Check sheet for the modelled part. Datum: model origin and axes. Units: mm. A direction names the side the tool comes from. Give positions to 0.01 mm unless a question says otherwise; leave off trailing zeros. Write each loop counter-clockwise with the first axis right and the second up, starting at its lowest first coordinate (ties: lowest second). Pieces come first, ordered by that corner, then holes. Notation, with made-up numbers: M -9.75,75 L 21.25,75 A21 cw 21.25,105 Z; hole C -21,54.5 d10. An arc over 180 degrees is marked long. Write item = value, one per line. Start each with the question number.
1) Sectioned sample at A-A, the plane z = -12. Record the cut outline in (x, y), then the cut area to 3 significant figures.
2) Scan lines: L1, parallel to X at y = 2.15, z = -4; L2, parallel to Z at x = 10.25, y = 1.5; L3, parallel to X at y = 0.3, z = -7.5. Record each from-to range of solid material in increasing order.
3) Gauge pin test, flat ends, axial feed: pin 1 (3 mm diameter, centred on x = 8, z = -10, fed in from +Y); pin 2 (0.5 mm diameter, centred on x = 12, z = -12, fed in from -Y); pin 3 (3 mm diameter, centred on x = 7, z = -3.5, fed in from -Y). Record the tip position at first contact, or that the pin passes through.
4) Draft check along X on faces 4 (the face through (4.78, 2.39, -11.83)), 5 (the face through (15, 0, -8)), 6 (the face through (4, 3.2, -4)), 7 (the face through (16, 2, -8)). Enter one of: pulls with the +X half, pulls with the -X half, needs draft (parallel to the pull), parting line crosses it, or undercut.
5) Sectioned sample at D-D, the plane y = 0.45. Record the cut outline in (x, z), then the cut area to 3 significant figures.
6) Sectioned sample at C-C, the plane x = 7.5. Record the cut outline in (y, z), then the cut area to 3 significant figures.
7) Set-up check for faces 1 (the face through (12, 4.8, -4)), 2 (the face through (3.28, 3.99, -6.29)), 3 (the face through (8, 1.6, -8)): record each of +Z, -Z, +X, -X, +Y, -Y from which the full face is reachable in a straight line by a thin tool's end or side.
8) Sectioned sample at B-B, the plane y = 2.5. Record the cut outline in (x, z), then the cut area to 3 significant figures.
from build123d import *

# Parameters (mm, degrees)
SKETCH1_W            = 16
SKETCH1_H            = 16
BOSS_EXTRUDE1_DEPTH  = 3.2
SKETCH2_R            = 2.4
BOSS_EXTRUDE2_DEPTH  = 1.6
LPATTERN1_COUNT      = 2
LPATTERN1_PITCH      = 8
LPATTERN1_COUNT_DIR2 = 4
LPATTERN1_PITCH_DIR2 = 8
SHELL1_T             = -1.6


with BuildPart() as part:
    # Sketch1 → Boss-Extrude1 (new body)
    with BuildSketch(Plane(origin=(0, 0, 0), x_dir=(1, 0, 0), z_dir=(0, 1, 0))):
        with Locations((8, 8)):
            Rectangle(SKETCH1_W, SKETCH1_H)
    extrude(amount=BOSS_EXTRUDE1_DEPTH)

    # Sketch2 → Boss-Extrude2 (add)
    with BuildSketch(Plane(origin=(0, 3.2, 0), x_dir=(1, 0, 0), z_dir=(0, 1, 0))):
        with Locations(Location((12, 4, 0), (0, 0, 90))):
            Circle(SKETCH2_R)
    boss_extrude2 = extrude(amount=BOSS_EXTRUDE2_DEPTH)

    # LPattern1: Boss-Extrude2 2 × 4, 4 skipped
    with Locations(*[(-i * LPATTERN1_PITCH, 0, -j * LPATTERN1_PITCH_DIR2) for i in range(LPATTERN1_COUNT) for j in range(LPATTERN1_COUNT_DIR2) if (i, j) not in ((0, 0), (0, 2), (0, 3), (1, 2), (1, 3))]):
        add(boss_extrude2)

    # Shell1
    shell1_openings = [part.faces().sort_by_distance(p)[0] for p in [
        (8, 0, -8),
    ]]
    offset(amount=SHELL1_T, openings=shell1_openings, kind=Kind.INTERSECTION)


solid = part.part
Data:
q1.outline = M 0,0 L 1.6,0 L 1.6,1.6 L 3.2,1.6 L 3.2,3.2 L 4.8,3.2 L 4.8,1.6 L 11.2,1.6 L 11.2,3.2 L 12.8,3.2 L 12.8,1.6 L 14.4,1.6 L 14.4,0 L 16,0 L 16,3.2 L 14.4,3.2 L 14.4,4.8 L 9.6,4.8 L 9.6,3.2 L 6.4,3.2 L 6.4,4.8 L 1.6,4.8 L 1.6,3.2 L 0,3.2 Z
q1.area = 41.0 mm2
q2.L1 = 0 to 3.2, 4.8 to 11.2, 12.8 to 16
q2.L2 = -16 to -14.4, -1.6 to 0
q2.L3 = 0 to 1.6, 14.4 to 16
q3.pin_1 = 3.2
q3.pin_2 = 3.2
q3.pin_3 = 1.6
q4.face_4 = undercut
q4.face_5 = needs draft
q4.face_6 = undercut
q4.face_7 = pulls with the +X half
q5.outline = M 0,-16 L 16,-16 L 16,0 L 0,0 Z; hole M 1.6,-14.4 L 14.4,-14.4 L 14.4,-1.6 L 1.6,-1.6 Z
q5.area = 92.2 mm2
q6.outline = M 0,-16 L 3.2,-16 L 3.2,0 L 0,0 L 0,-1.6 L 1.6,-1.6 L 1.6,-14.4 L 0,-14.4 Z
q6.area = 30.7 mm2
q7.face_1 = +Z, -Z, +X, -X, +Y
q7.face_2 = +Y
q7.face_3 = -Y
q8.outline = M 0,-16 L 16,-16 L 16,0 L 0,0 Z; hole C 4,-12 d1.6; hole C 4,-4 d1.6; hole C 12,-12 d1.6; hole C 12,-4 d1.6
q8.area = 248 mm2
